Model file for the job. Use its own axes, mm. Coordinates: 2 decimals unless noted, no trailing zeros. Loops run counter-clockwise (first coordinate to the right, second up) from the corner with the lowest first, then second, coordinate; pieces in that order, holes last. Notation, with made-up numbers: M -1.5,18 L 25.5,18 A27 ccw 25.5,48 Z; hole C -27.5,52.5 d5. An arc over 180 degrees is marked long. One line per question, with ' | ' between items. Start each with the question number.
```python
from build123d import *

# Parameters (mm, degrees)
BOSS_EXTRUDE1_DEPTH      = 47.625
BOSS_EXTRUDE1_DEPTH_BACK = 2.54
SKETCH1_R                = 36.426767544
SKETCH4_R                = 4.7625
CUT_EXTRUDE1_DEPTH       = 139.904833197


with BuildPart() as part:
    # Sketch1 → Boss-Extrude1 (new, two sides: drawn at the far end of the back side and taken through both)
    with BuildSketch(Plane.XY.offset(-BOSS_EXTRUDE1_DEPTH_BACK)):
        with Locations((67.114492883, 307.327144707)):
            Circle(SKETCH1_R)
    extrude(amount=BOSS_EXTRUDE1_DEPTH + BOSS_EXTRUDE1_DEPTH_BACK)

    # Sketch3 → Revolve1 (revolve)
    with BuildSketch(Plane(origin=(67.114492883, 0, 0), x_dir=(0, 0, -1), z_dir=(1, 0, 0)), mode=Mode.PRIVATE) as revolve1_sk:
        with BuildLine():
            Line((-47.625, 307.327144707), (-57.15, 307.327144707))
            ThreePointArc((-57.15, 307.327144707), (-54.72938109, 326.152891828), (-47.625, 343.75391225))
            Line((-47.625, 343.75391225), (-47.625, 307.327144707))
        make_face()
        with BuildLine():
            Line((2.54, 307.327144707), (12.065, 307.327144707))
            ThreePointArc((12.065, 307.327144707), (9.64438109, 326.152891828), (2.54, 343.75391225))
            Line((2.54, 343.75391225), (2.54, 307.327144707))
        make_face()
    revolve(revolve1_sk.sketch.rotate(Axis((67.114492883, 307.327144707, 47.625), (0, 0, 1)), 90), axis=Axis((67.114492883, 307.327144707, 47.625), (0, 0, 1)))

    # Sketch4 → Cut-Extrude1 (cut, through all)
    with BuildSketch(Plane(origin=(0, 343.75391225, 0), x_dir=(1, 0, 0), z_dir=(0, 1, 0))):
        with Locations(Location((67.114492883, -22.225, 0), (0, 0, 270))):
            Circle(SKETCH4_R)
    extrude(amount=-CUT_EXTRUDE1_DEPTH, mode=Mode.SUBTRACT)


solid = part.part
```
(1) Band-saw the part on B-B on y = 329.5. Write the cut outline in (x, z) (1 decimal).
(2) Band-saw the part on D-D on y = 294. Write the cut outline in (x, z) (1 decimal).
(3) Drill centre lines: line 1 (X direction, y = 332, z = 18.5); line 2 (X direction, y = 290.5, z = 26); line 3 (Z direction, x = 65, y = 282.5). Where is each one in solid material? Low to high. Write a range as [from, to].
(4) Two-plate mould, pull along X, no slides. Class faces 1 (the face through (59.218, 271.767, 22.191)), 2 (the face through (71.836, 307.837, 21.605)): pulls with the +X half, pulls with the -X half, needs draft (parallel to the pull), parting line crosses it, or undercut.
(5) Pin check, flat tips, straight feed: P1, Ø1.5, axis at x = 48.5, y = 311, coming from the -Z side; P2, Ø6, axis at x = 50.5, z = 6.5, coming from the +Y side; P3, Ø12, axis at x = 84.5, z = 2.5, coming from the +Y side; P4, Ø15, axis at x = 67.11, z = 22.22, coming from the -Y side. Stop position of each tip, or through.
(6) Band-saw the part on C-C on z = 21. Write the cut outline in (x, y), then the cut area to 3 significant figures.
(7) Band-saw the part on A-A on x = 63.5. Write the cut outline in (y, z) (3 decimals).
Computed values:
1) outline: M 38.2,-2.5 A71 ccw 96,-2.5 L 96,47.6 A71 ccw 38.2,47.6 Z; hole C 67.1,22.2 d9.5
2) outline: M 33.2,-2.5 A73.2 ccw 101,-2.5 L 101,47.6 A73.2 ccw 33.2,47.6 Z; hole C 67.1,22.2 d9.5
3) line 1: [40.32, 64.15], [70.08, 93.91] | line 2: [34.81, 64.21], [70.02, 99.42] | line 3: [-7.77, 17.96], [26.49, 52.85]
4) face 1: parting line crosses it | face 2: undercut
5) P1: z = -9.8 | P2: y = 341.11 | P3: y = 341.93 | P4: y = 270.9
6) outline: M 62.51,271.19 L 62.51,343.46 A36.43 ccw Z; M 71.72,271.19 A36.43 ccw 71.72,343.46 Z | area: 3,500 mm^2
7) outline: M 271.08,-2.54 A74.329 ccw 343.574,-2.54 L 343.574,19.124 L 271.08,19.124 Z; M 271.08,25.326 L 343.574,25.326 L 343.574,47.625 A74.329 ccw 271.08,47.625 Z
